```python
from build123d import *

# Parameters (mm, degrees)
BOSS_EXTRUDE1_DEPTH  = 100
BOSS_EXTRUDE2_DEPTH  = 10
BOSS_EXTRUDE2_DRAFT  = 45
SKETCH4_R            = 34.5
BOSS_EXTRUDE3_DEPTH  = 10
SKETCH5_R            = 31
BOSS_EXTRUDE4_DEPTH  = 30
SKETCH6_R            = 2.5
SKETCH6_R_2          = 1.5
BOSS_EXTRUDE5_DEPTH  = 1
CIRPATTERN1_COUNT    = 12
BOSS_EXTRUDE6_DEPTH  = 100
SKETCH8_R            = 31
BOSS_EXTRUDE7_DEPTH  = 10
SKETCH9_R            = 30
BOSS_EXTRUDE8_DEPTH  = 1
SKETCH10_R           = 31
BOSS_EXTRUDE9_DEPTH  = 10
SKETCH11_R           = 42.5
BOSS_EXTRUDE10_DEPTH = 10.5
BOSS_EXTRUDE11_DEPTH = 35
BOSS_EXTRUDE12_DEPTH = 40
CUT_EXTRUDE1_DEPTH   = 40
SKETCH15_R           = 15
CUT_EXTRUDE2_DEPTH   = 20
SKETCH16_R           = 15
CUT_EXTRUDE3_DEPTH   = 20


with BuildPart() as part:
    # Sketch1 → Boss-Extrude1 (new body)
    with BuildSketch(Plane(origin=(0, 0, 0), x_dir=(0, 0, -1), z_dir=(1, 0, 0))):
        with BuildLine():
            Line((-37.5, 45), (37.5, 45))
            ThreePointArc((37.5, 45), (45.880962103, 0), (37.5, -45))
            Line((37.5, -45), (-37.5, -45))
            ThreePointArc((-37.5, -45), (-45.880962103, 0), (-37.5, 45))
        make_face()
    extrude(amount=BOSS_EXTRUDE1_DEPTH)


with BuildPart() as boss_extrude2_tool:
    # Sketch2 → Boss-Extrude2 (with draft: the straight prism first)
    with BuildSketch(Plane(origin=(100, 0, 0), x_dir=(0, 0, -1), z_dir=(1, 0, 0))):
        with BuildLine():
            Line((37.5, 45), (-37.5, 45))
            ThreePointArc((-37.5, 45), (-45.880962103, 0), (-37.5, -45))
            Line((-37.5, -45), (37.5, -45))
            ThreePointArc((37.5, -45), (45.880962103, 0), (37.5, 45))
        make_face()
    extrude(amount=BOSS_EXTRUDE2_DEPTH)
    # Boss-Extrude2: the draft: its side faces are tilted about the plane it starts from
    boss_extrude2_sides = [boss_extrude2_tool.faces().sort_by_distance(p)[0] for p in [
        (105, -45, 0),
        (105, 0, -45.880962103),
        (105, 45, 0),
        (105, 0, 45.880962103),
    ]]
    draft(boss_extrude2_sides, Plane(origin=(100, 0, 0), x_dir=(0, 0, -1), z_dir=(1, 0, 0)), BOSS_EXTRUDE2_DRAFT)


with BuildPart() as part_1:
    add(part.part)

    # Boss-Extrude2: add boss_extrude2_tool
    add(boss_extrude2_tool.part)

    # Sketch4 → Boss-Extrude3 (add)
    with BuildSketch(Plane(origin=(110, 0, 0), x_dir=(0, 0, -1), z_dir=(1, 0, 0))):
        Circle(SKETCH4_R)
    extrude(amount=BOSS_EXTRUDE3_DEPTH)

    # Sketch5 → Boss-Extrude4 (add)
    with BuildSketch(Plane(origin=(120, 0, 0), x_dir=(0, 0, -1), z_dir=(1, 0, 0))):
        Circle(SKETCH5_R)
    extrude(amount=BOSS_EXTRUDE4_DEPTH)

    # Sketch6 → Boss-Extrude5 (add)
    with BuildSketch(Plane(origin=(150, 0, 0), x_dir=(0, 0, -1), z_dir=(1, 0, 0))):
        with Locations((27, 0)):
            Circle(SKETCH6_R)
        with Locations((27, 0)):
            Circle(SKETCH6_R_2, mode=Mode.SUBTRACT)
    boss_extrude5 = extrude(amount=BOSS_EXTRUDE5_DEPTH)

    # CirPattern1: Boss-Extrude5 ×12 about axis
    cirpattern1_axis = Axis((0, 0, 0.17674784), (1, 0, 0))
    for i in range(1, CIRPATTERN1_COUNT):
        add(boss_extrude5.rotate(cirpattern1_axis, i * 360 / CIRPATTERN1_COUNT))

    # Sketch7 → Boss-Extrude6 (add)
    with BuildSketch(Plane(origin=(150, 0, 0), x_dir=(0, 0, -1), z_dir=(1, 0, 0))):
        with BuildLine():
            Line((16, 17), (16, -17))
            ThreePointArc((16, -17), (0, -23.900331129), (-16, -17))
            Line((-16, -17), (-16, 17))
            ThreePointArc((-16, 17), (0, 23.900331129), (16, 17))
        make_face()
    extrude(amount=BOSS_EXTRUDE6_DEPTH)

    # Sketch8 → Boss-Extrude7 (add)
    with BuildSketch(Plane(origin=(250, 0, 0), x_dir=(0, 0, -1), z_dir=(1, 0, 0))):
        Circle(SKETCH8_R)
    extrude(amount=BOSS_EXTRUDE7_DEPTH)

    # Sketch9 → Boss-Extrude8 (add)
    with BuildSketch(Plane(origin=(260, 0, 0), x_dir=(0, 0, -1), z_dir=(1, 0, 0))):
        Circle(SKETCH9_R)
    extrude(amount=BOSS_EXTRUDE8_DEPTH)

    # Sketch10 → Boss-Extrude9 (add)
    with BuildSketch(Plane(origin=(261, 0, 0), x_dir=(0, 0, -1), z_dir=(1, 0, 0))):
        Circle(SKETCH10_R)
    extrude(amount=BOSS_EXTRUDE9_DEPTH)

    # Sketch11 → Boss-Extrude10 (add, symmetric)
    with BuildSketch(Plane.XY.offset(37.5)):
        with Locations((50, -45)):
            Circle(SKETCH11_R)
    extrude(amount=BOSS_EXTRUDE10_DEPTH, both=True)

    # Sketch12 → Boss-Extrude11 (add)
    with BuildSketch(Plane(origin=(0, 0, 27), x_dir=(-1, 0, 0), z_dir=(0, 0, -1))):
        with BuildLine():
            Line((-68.570979575, -45), (-28.570979575, -45))
            Line((-28.570979575, -45), (-28.570979575, -75))
            ThreePointArc((-28.570979575, -75), (-48.570979575, -82.639320225), (-68.570979575, -75))
            Line((-68.570979575, -75), (-68.570979575, -45))
        make_face()
    extrude(amount=BOSS_EXTRUDE11_DEPTH)

    # Sketch13 → Boss-Extrude12 (add)
    with BuildSketch(Plane(origin=(68.570979575, 0, 0), x_dir=(0, 0, -1), z_dir=(1, 0, 0))):
        with BuildLine():
            Line((8, -45), (8, -87))
            ThreePointArc((8, -87), (25.421855105, -68.929675658), (33, -45))
            Line((33, -45), (8, -45))
        make_face()
    extrude(amount=-BOSS_EXTRUDE12_DEPTH)

    # Sketch14 → Cut-Extrude1 (cut)
    with BuildSketch(Plane.XY.offset(-8)):
        with BuildLine():
            Line((28.570979575, -75), (28.570979575, -87))
            Line((28.570979575, -87), (68.570979575, -87))
            Line((68.570979575, -87), (68.570979575, -75))
            ThreePointArc((68.570979575, -75), (48.570979575, -82.639320225), (28.570979575, -75))
        make_face()
    extrude(amount=-CUT_EXTRUDE1_DEPTH, mode=Mode.SUBTRACT)

    # Sketch15 → Cut-Extrude2 (cut)
    with BuildSketch(Plane(origin=(271, 0, 0), x_dir=(0, 0, -1), z_dir=(1, 0, 0))):
        Circle(SKETCH15_R)
    extrude(amount=-CUT_EXTRUDE2_DEPTH, mode=Mode.SUBTRACT)

    # Sketch16 → Cut-Extrude3 (cut)
    with BuildSketch(Plane.XY.offset(48)):
        with Locations((50, -45)):
            Circle(SKETCH16_R)
    extrude(amount=-CUT_EXTRUDE3_DEPTH, mode=Mode.SUBTRACT)


solid = part_1.part
```
Verification items for the finished model (mm, model axes). A direction names the side the tool comes from. Coordinates: 2 decimals unless noted, no trailing zeros. Loops run counter-clockwise (first coordinate to the right, second up) from the corner with the lowest first, then second, coordinate; pieces in that order, holes last. Notation, with made-up numbers: (39.25, 22.25) -> (96.25, 22.25) arc R10 ccw to (96.25, 27.25) -> close; hole circle Ø4 at (86.5, 66.25). An arc over 180 degrees is marked (long way). Put each result on its own line as item: value.
1. Gauge pin test, flat ends, axial feed: P1, Ø5, axis at x = 203, y = 16, coming from the +Z side; P2, Ø4, axis at x = 204.5, z = 16, coming from the +Y side; P3, Ø6, axis at x = 119, z = -12, coming from the +Y side. Record the tip position at first contact, or that the pin passes through.
Result set:
P1: stops at z = 16
P2: stops at y = 18.87
P3: stops at y = 33.31
2. Tool access check on faces 1 (the face through (151, 2, 27)), 2 (the face through (134.79, 30.736, 4.036)), 3 (the face through (151, -25, 15)), 4 (the face through (250, 0, -20)), 5 (the face through (151, -27, 2)). Record the directions out of +Z, -Z, +X, -X, +Y, -Y that give a thin tool (end or side, any length) a straight path to the whole face; none if there is none.
Result set:
face 1: +Z, +Y, -Y
face 2: +X
face 3: +Z, -Y
face 4: none
face 5: +Z, -Z, -Y
3. Section check D-D, the plane x = 137. Record the boundary of the cut face in (y, z), then the cut area to 3 significant figures.
Result set:
outline: circle Ø62 at (0, 0)
area: 3,020 mm^2
4. Mould release check, pull along X, two halves, no side actions. Record for faces 6 (the face through (151, 0, -29)), 7 (the face through (106.04, 0.61, 39.84)), 8 (the face through (69, -65, 27)): pulls with the +X half, pulls with the -X half, needs draft (parallel to the pull), parting line crosses it, or undercut.
Result set:
face 6: undercut
face 7: pulls with the +X half
face 8: needs draft
5. Section check C-C, the plane x = 50. Record the boundary of the cut face in (y, z).
Result set:
outline: (-87.5, 27) -> (-82.61, 27) -> (-82.61, -13.9) arc R55 ccw to (-45, -33) -> (-45, -37.5) arc R125 ccw to (45, -37.5) -> (45, 37.5) arc R125 ccw to (-2.5, 45.86) -> (-2.5, 48) -> (-30, 48) -> (-30, 28) -> (-60, 28) -> (-60, 48) -> (-87.5, 48) -> close
6. Section check A-A, the plane x = 216. Record the boundary of the cut face in (y, z).
Result set:
outline: (-17, -16) -> (17, -16) arc R22 ccw to (17, 16) -> (-17, 16) arc R22 ccw to start
7. Section check B-B, the plane y = -55. Record the boundary of the cut face in (x, z).
Result set:
outline: (8.69, 27) -> (28.57, 27) -> (28.57, -31.3) -> (68.57, -31.3) -> (68.57, 27) -> (91.31, 27) -> (91.31, 48) -> (61.18, 48) -> (61.18, 28) -> (38.82, 28) -> (38.82, 48) -> (8.69, 48) -> close
8. Thickness scan on line 1 (X direction, y = -13, z = -21); line 2 (Y direction, x = 84.5, z = -24); line 3 (X direction, y = -58, z = -21). Record the ranges inside material, lowest first.
Result set:
line 1: x = 0 to 151, 250 to 271
line 2: y = -45 to 45
line 3: x = 28.57 to 68.57
